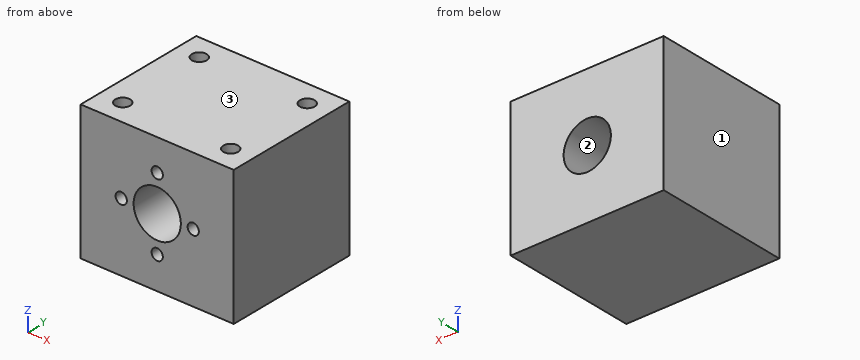
from build123d import *

# Parameters (mm, degrees)
SKETCH495_W       = 34
SKETCH495_H       = 30.2
PAD219_DEPTH      = 15
PAD219_DEPTH_BACK = 15.2
SKETCH726_R       = 1.65
HOLE001_DEPTH     = 20
HOLE001_TIPS_R    = 1.65
SKETCH727_R       = 5.25
POCKET255_DEPTH   = 30.2
SKETCH728_R       = 1.25
HOLE002_DEPTH     = 15
HOLE002_TIPS_R    = 1.25


with BuildPart() as part:
    # Sketch495 → Pad219 (new body, two sides)
    with BuildSketch(Plane.XY) as pad219_sk:
        Rectangle(SKETCH495_W, SKETCH495_H)
    extrude(amount=PAD219_DEPTH)
    extrude(pad219_sk.sketch, amount=-PAD219_DEPTH_BACK)

    # Sketch726 (on Face6 of Pad219) → Hole001 (cut)
    with BuildSketch(Plane.XY.offset(15)):
        with Locations((-12, 10)):
            Circle(SKETCH726_R)
        with Locations((12, 10)):
            Circle(SKETCH726_R)
        with Locations((12, -10)):
            Circle(SKETCH726_R)
        with Locations((-12, -10)):
            Circle(SKETCH726_R)
    extrude(amount=-HOLE001_DEPTH, mode=Mode.SUBTRACT)

    # Hole001 tips → Hole001 tip 1 section 0
    with BuildSketch(Plane.XY.offset(-5), mode=Mode.PRIVATE) as hole001_tip_1_s0:
        with Locations((-12, 10)):
            Circle(HOLE001_TIPS_R)
    loft([hole001_tip_1_s0.sketch, Vertex(-12, 10, -5.99142)], mode=Mode.SUBTRACT)

    # Hole001 tips → Hole001 tip 2 section 0
    with BuildSketch(Plane.XY.offset(-5), mode=Mode.PRIVATE) as hole001_tip_2_s0:
        with Locations((12, 10)):
            Circle(HOLE001_TIPS_R)
    loft([hole001_tip_2_s0.sketch, Vertex(12, 10, -5.99142)], mode=Mode.SUBTRACT)

    # Hole001 tips → Hole001 tip 3 section 0
    with BuildSketch(Plane.XY.offset(-5), mode=Mode.PRIVATE) as hole001_tip_3_s0:
        with Locations((12, -10)):
            Circle(HOLE001_TIPS_R)
    loft([hole001_tip_3_s0.sketch, Vertex(12, -10, -5.99142)], mode=Mode.SUBTRACT)

    # Hole001 tips → Hole001 tip 4 section 0
    with BuildSketch(Plane.XY.offset(-5), mode=Mode.PRIVATE) as hole001_tip_4_s0:
        with Locations((-12, -10)):
            Circle(HOLE001_TIPS_R)
    loft([hole001_tip_4_s0.sketch, Vertex(-12, -10, -5.99142)], mode=Mode.SUBTRACT)

    # Sketch727 (on Face3 of Hole001) → Pocket255 (cut)
    with BuildSketch(Plane.XZ.offset(15.1)):
        Circle(SKETCH727_R)
    extrude(amount=-POCKET255_DEPTH, mode=Mode.SUBTRACT)

    # Sketch728 (on Face3 of Pocket255) → Hole002 (cut)
    with BuildSketch(Plane.XZ.offset(15.1)):
        with Locations((0, 8)):
            Circle(SKETCH728_R)
        with Locations((8, 0)):
            Circle(SKETCH728_R)
        with Locations((0, -8)):
            Circle(SKETCH728_R)
        with Locations((-8, 0)):
            Circle(SKETCH728_R)
    extrude(amount=-HOLE002_DEPTH, mode=Mode.SUBTRACT)

    # Hole002 tips → Hole002 tip 1 section 0
    with BuildSketch(Plane.XZ.offset(0.1), mode=Mode.PRIVATE) as hole002_tip_1_s0:
        with Locations((0, 8)):
            Circle(HOLE002_TIPS_R)
    loft([hole002_tip_1_s0.sketch, Vertex(0, 0.651076, 8)], mode=Mode.SUBTRACT)

    # Hole002 tips → Hole002 tip 2 section 0
    with BuildSketch(Plane.XZ.offset(0.1), mode=Mode.PRIVATE) as hole002_tip_2_s0:
        with Locations((8, 0)):
            Circle(HOLE002_TIPS_R)
    loft([hole002_tip_2_s0.sketch, Vertex(8, 0.651076, 0)], mode=Mode.SUBTRACT)

    # Hole002 tips → Hole002 tip 3 section 0
    with BuildSketch(Plane.XZ.offset(0.1), mode=Mode.PRIVATE) as hole002_tip_3_s0:
        with Locations((0, -8)):
            Circle(HOLE002_TIPS_R)
    loft([hole002_tip_3_s0.sketch, Vertex(0, 0.651076, -8)], mode=Mode.SUBTRACT)

    # Hole002 tips → Hole002 tip 4 section 0
    with BuildSketch(Plane.XZ.offset(0.1), mode=Mode.PRIVATE) as hole002_tip_4_s0:
        with Locations((-8, 0)):
            Circle(HOLE002_TIPS_R)
    loft([hole002_tip_4_s0.sketch, Vertex(-8, 0.651076, 0)], mode=Mode.SUBTRACT)


with BuildPart() as part_1:
    # Body150 placement: moved
    add(part.part.moved(Location((0, 0, 16))))


solid = part_1.part
Model file for the job. Use its own axes, mm. Face numbers are marked on the shaded views. Round coordinates to 2 decimals unless told otherwise and drop trailing zeros. Order: outer loops, then holes, each group sorted by start corner. A loop starts at its lowest first (then second) coordinate and runs counter-clockwise, first axis right, second up.
(1) Pull direction X, two halves, no side cores. Call the marked faces 1, 2 and 3: released by +X, released by -X, zero draft, split by the parting line, or undercut.
(2) Band-saw the part on B-B (x = -3). List the corners of the cut face in (y, z), then the cut area to 3 significant figures.
(3) Band-saw the part on A-A (z = 11.5). List the corners of the cut face in (x, y).
(4) Band-saw the part on C-C (y = -7.5). List the corners of the cut face in (x, z), then the cut area to 3 significant figures.
(5) Drill centre lines: line 1 (Z direction, x = 0, y = -4); line 2 (Y direction, x = -12, z = 23.25); line 3 (Z direction, x = 1, y = -1). Where is each one in solid material? Low to high.
(6) Band-saw the part on D-D (y = 3). List the corners of the cut face in (x, z), then the cut area to 3 significant figures.
(7) Pin check, flat tips, straight feed: pin 1 (2 mm diameter, centred on x = 0, z = 24, fed in from -Y); pin 2 (1.5 mm diameter, centred on x = 0, z = 8, fed in from -Y). Stop position of each tip, or through.
Verdict:
1. face 1: released by -X
1. face 2: undercut
1. face 3: zero draft
2. outline: (-15.1, 0.8) - (15.1, 0.8) - (15.1, 11.69) - (-15.1, 11.69) - close; (-15.1, 20.31) - (15.1, 20.31) - (15.1, 31) - (-15.1, 31) - close
2. area: 652 mm2
3. outline: (-17, -15.1) - (-2.7, -15.1) - (-2.7, 15.1) - (-17, 15.1) - close; (2.7, -15.1) - (17, -15.1) - (17, 15.1) - (2.7, 15.1) - close; hole circle Ø3.3 at (-12, -10); hole circle Ø3.3 at (-12, 10); hole circle Ø3.3 at (12, -10); hole circle Ø3.3 at (12, 10)
4. outline: (-17, 0.8) - (17, 0.8) - (17, 31) - (-17, 31) - close; hole circle Ø2.5 at (-8, 16); hole circle Ø10.5 at (0, 16); hole circle Ø2.5 at (0, 8); hole circle Ø2.5 at (0, 24); hole circle Ø2.5 at (8, 16)
4. area: 921 mm2
5. line 1: z = 0.8 to 6.75, 9.25 to 10.75, 21.25 to 22.75, 25.25 to 31
5. line 2: y = -15.1 to -11.65, -8.35 to 8.35, 11.65 to 15.1
5. line 3: z = 0.8 to 7.25, 8.75 to 10.85, 21.15 to 23.25, 24.75 to 31
6. outline: (-17, 0.8) - (17, 0.8) - (17, 31) - (-17, 31) - close; hole circle Ø10.5 at (0, 16)
6. area: 940 mm2
7. pin 1: stops at y = 0.05
7. pin 2: stops at y = 0.2
